Here's how the part is built. I have some questions about the finished solid (model axes, mm). Face numbers are marked on the shaded views. A direction names the side the tool comes from. Coordinates: 2 decimals unless noted, no trailing zeros. Write each loop counter-clockwise with the first axis right and the second up, starting at its lowest first coordinate (ties: lowest second). Pieces come first, ordered by that corner, then holes. Notation, with made-up numbers: M 85,85.5 L 132,85.5 A27 ccw 132,116.5 Z; hole C 56.5,67.5 d7. An arc over 180 degrees is marked long. Use a Markdown table: item, result.
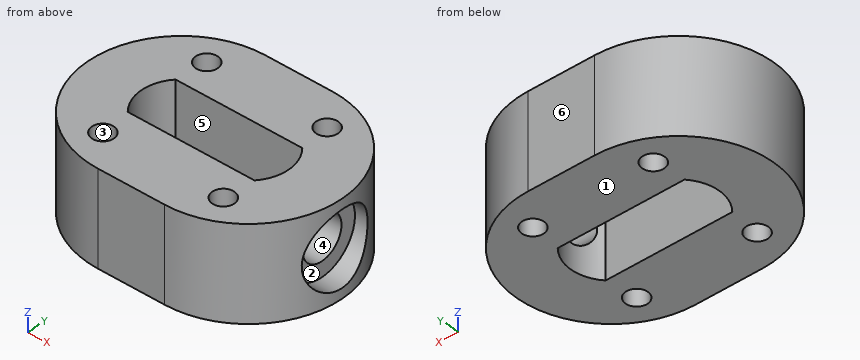
```python
from build123d import *

# Parameters (mm, degrees)
BOSS_EXTRUDE1_DEPTH     = 14
M4_TAPPED_HOLE2_D       = 3.3
CUT_EXTRUDE1_REACH      = 44.849
CUT_EXTRUDE1_END_RADIUS = 6
SKETCH5_R               = 3.25
SKETCH6_R               = 5.5
CUT_EXTRUDE2_DEPTH      = 3


with BuildPart() as part:
    # Sketch1 → Boss-Extrude1 (new body)
    with BuildSketch(Plane.XY):
        with BuildLine():
            Line((0, 14), (10, 14))
            ThreePointArc((10, 14), (24, 0), (10, -14))
            Line((10, -14), (0, -14))
            ThreePointArc((0, -14), (-14, 0), (0, 14))
        make_face()
        with BuildLine():
            Line((-4.472135955, 4), (14.472135955, 4))
            ThreePointArc((14.472135955, 4), (16, 0), (14.472135955, -4))
            Line((14.472135955, -4), (-4.472135955, -4))
            ThreePointArc((-4.472135955, -4), (-6, 0), (-4.472135955, 4))
        make_face(mode=Mode.SUBTRACT)
    extrude(amount=BOSS_EXTRUDE1_DEPTH)

    # M4 Tapped Hole2 (through all)
    with Locations(Plane(origin=(-3.996947905, 8.674675786, 14), x_dir=(1, 0, 0), z_dir=(0, 0, 1))):
        with Locations((0, 0), (18, 0), (18, -17.349351572), (0, -17.349351572)):
            Hole(M4_TAPPED_HOLE2_D / 2)

    # Cut-Extrude1: up to this cylinder (the profile starts outside it)
    cut_extrude1_end = Plane(origin=(10, 0, 7), z_dir=(0, 0, -1)) * Cylinder(CUT_EXTRUDE1_END_RADIUS, 102.698, mode=Mode.PRIVATE)
    # Sketch5 → Cut-Extrude1 (cut, up to the surface)
    with BuildSketch(Plane(origin=(24, 0, 0), x_dir=(0, 0, -1), z_dir=(1, 0, 0)), mode=Mode.PRIVATE) as cut_extrude1_sk1:
        with Locations((-7, 0)):
            Circle(SKETCH5_R)
    cut_extrude1_tool1 = extrude(cut_extrude1_sk1.sketch, amount=-CUT_EXTRUDE1_REACH, mode=Mode.PRIVATE) - cut_extrude1_end
    add(cut_extrude1_tool1.solids().sort_by_distance((24, 0, 7))[0], mode=Mode.SUBTRACT)

    # Sketch6 → Cut-Extrude2 (cut)
    with BuildSketch(Plane(origin=(24, 0, 0), x_dir=(0, 0, -1), z_dir=(1, 0, 0))):
        with Locations((-7, 0)):
            Circle(SKETCH6_R)
    extrude(amount=-CUT_EXTRUDE2_DEPTH, mode=Mode.SUBTRACT)


solid = part.part
```
1. Suppose I cut it at A-A on x = 3.5. Write out the boundary of the cut face in (y, z), and give its area (3 significant figures).
Answers follow:
| item | result |
|---|---|
| outline | M -14,0 L -4,0 L -4,14 L -14,14 Z; M 4,0 L 14,0 L 14,14 L 4,14 Z |
| area | 280 mm2 |
2. Which directions (+Z, -Z, +X, -X, +Y, -Y) give clear straight access to the entire face, cutting with the end or side of a thin tool? Please do the marked faces 4, 5 and 6.
Answers follow:
| item | result |
|---|---|
| face 4 | +X |
| face 5 | +Z, -Z |
| face 6 | +Z, -Z, +X, -X, +Y |
3. Will these pins go through, and if not, where does the flat tip stop? pin 1 Ø2 at (x, z) = (18.5, 4) entering from +Y; pin 2 Ø6 at (y, z) = (2.5, 4.5) entering from +X; pin 3 Ø5.5 at (x, y) = (-4, 8.67) entering from +Z; pin 4 Ø5 at (y, z) = (0, 7) entering from +X.
Answers follow:
| item | result |
|---|---|
| pin 1 | stops at y = 11.82 |
| pin 2 | stops at x = 23.93 |
| pin 3 | stops at z = 14 |
| pin 4 | stops at x = -5.45 |
4. Suppose I cut it at B-B on y = 0. Write out the boundary of the cut face in (x, z).
Answers follow:
| item | result |
|---|---|
| outline | M -14,0 L -6,0 L -6,14 L -14,14 Z; M 16,0 L 24,0 L 24,1.5 L 21,1.5 L 21,3.75 L 16,3.75 Z; M 16,10.25 L 21,10.25 L 21,12.5 L 24,12.5 L 24,14 L 16,14 Z |
5. I need wall thicknesses on probe 1 along Y at (x, z) = (3.5, 11); probe 2 along X at (y, z) = (9.25, 10.5); probe 3 along Z at (x, y) = (19.85, 0). Which ranges of each line are inside material? Lowest first, please.
Answers follow:
| item | result |
|---|---|
| probe 1 | y = -14 to -4, 4 to 14 |
| probe 2 | x = -10.51 to -5.54, -2.45 to 12.46, 15.55 to 20.51 |
| probe 3 | z = 0 to 3.75, 10.25 to 14 |
6. We'd pull the mould along Z, two halves only. Please class the marked faces 1, 2 and 3: +Z half, -Z half, draft (parallel to the pull), parting line (faces both ways), or undercut.
Answers follow:
| item | result |
|---|---|
| face 1 | -Z half |
| face 2 | undercut |
| face 3 | draft |
7. Suppose I cut it at C-C on z = 9.25. Write out the boundary of the cut face in (x, y), and give its area (3 significant figures).
Answers follow:
| item | result |
|---|---|
| outline | M -4.47,-4 A6 cw -4.47,4 L 14.47,4 A6 cw 15.52,2.35 L 21,2.35 L 21,5.02 L 23.07,5.02 A14 ccw 10,14 L 0,14 A14 ccw 0,-14 L 10,-14 A14 ccw 23.07,-5.02 L 21,-5.02 L 21,-2.35 L 15.52,-2.35 A6 cw 14.47,-4 Z; hole C -4,-8.67 d3.3; hole C -4,8.67 d3.3; hole C 14,-8.67 d3.3; hole C 14,8.67 d3.3 |
| area | 642 mm2 |
8. Suppose I cut it at D-D on z = 11.75. Write out the boundary of the cut face in (x, y).
Answers follow:
| item | result |
|---|---|
| outline | M 0,-14 L 10,-14 A14 ccw 23.72,-2.77 L 21,-2.77 L 21,2.77 L 23.72,2.77 A14 ccw 10,14 L 0,14 A14 ccw Z; hole C -4,-8.67 d3.3; hole C -4,8.67 d3.3; hole M -4.47,-4 L 14.47,-4 A6 ccw 14.47,4 L -4.47,4 A6 ccw Z; hole C 14,-8.67 d3.3; hole C 14,8.67 d3.3 |
